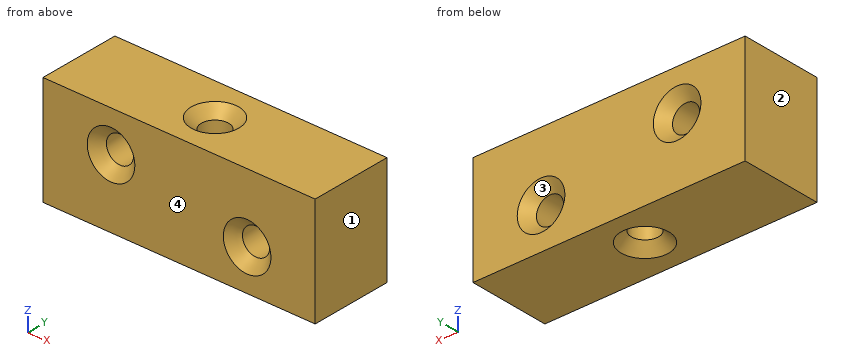
```python
from build123d import *

# Parameters (mm, degrees)
F0_W     = 40
F0_H     = 16
F0_R     = 2
F1_DEPTH = 12
F2_R     = 2
F3_DEPTH = 16.001
F4_SIZE  = 1.5


with BuildPart() as f1:
    # F0 (on Front) → F1 (new body)
    with BuildSketch(Plane.XZ):
        Rectangle(F0_W, F0_H)
        with Locations((10, -2)):
            Circle(F0_R, mode=Mode.SUBTRACT)
        with Locations((-10, 2)):
            Circle(F0_R, mode=Mode.SUBTRACT)
    extrude(amount=-F1_DEPTH)

    # F2 (on face) → F3 (cut, through all)
    with BuildSketch(Plane.XY.offset(8)):
        with Locations((0, 6)):
            Circle(F2_R)
    extrude(amount=-F3_DEPTH, mode=Mode.SUBTRACT)

    # F4
    f4_edges = [f1.edges().sort_by_distance(p)[0] for p in [
        (-12, 12, 2),
        (8, 12, -2),
        (-12, 0, 2),
        (8, 0, -2),
        (-2, 6, 8),
        (-2, 6, -8),
    ]]
    chamfer(f4_edges, length=F4_SIZE)


solid = f1.part
```
Can you work these out from the model? Positions are in its coordinate system, mm. Face numbers are marked on the shaded views. Coordinates: 2 decimals unless noted, no trailing zeros. Order: outer loops, then holes, each group sorted by start corner. A loop starts at its lowest first (then second) coordinate and runs counter-clockwise, first axis right, second up.
1. I need wall thicknesses on line 1 (Z direction, x = -10, y = 3.75); line 2 (Z direction, x = 10, y = 4.5); line 3 (X direction, y = 5.5, z = -2.5). Which ranges of each line are inside material? Lowest first, please.
2. If we section it at A-A (y = 6): Please give me the cut outline in (x, z), then the cut area to 3 significant figures.
3. If we section it at D-D (z = 6): Please give me the cut outline in (x, y), then the cut area to 3 significant figures.
4. Thinking about a two-plate mould opening in X: for the marked faces 1, 2, 3 and 4, which applies, +X half, -X half, draft (parallel to the pull), parting line (faces both ways), or undercut?
5. I'm going to push flat-ended pins straight in: pin 1 (8 mm diameter, centred on x = 14, z = 5.5, fed in from -Y); pin 2 (5 mm diameter, centred on x = -10, z = 2, fed in from +Y). Where does each tip first touch, or does it pass through?
6. If we section it at B-B (x = 0): Please give me the cut outline in (y, z).
7. If we section it at C-C (z = -2): Please give me the cut outline in (x, y), then the cut area to 3 significant figures.
Entries:
1. line 1: z = -8 to 0, 4 to 8
1. line 2: z = -8 to -4, 0 to 8
1. line 3: x = -20 to -1.94, 1.94 to 8.06, 11.94 to 20
2. outline: (-20, -8) - (-3.5, -8) - (-2, -6.5) - (-2, 6.5) - (-3.5, 8) - (-20, 8) - close; (2, -6.5) - (3.5, -8) - (20, -8) - (20, 8) - (3.5, 8) - (2, 6.5) - close; hole circle Ø4 at (-10, 2); hole circle Ø4 at (10, -2)
2. area: 546 mm2
3. outline: (-20, 0) - (20, 0) - (20, 12) - (-20, 12) - close; hole circle Ø4 at (0, 6)
3. area: 467 mm2
4. face 1: +X half
4. face 2: -X half
4. face 3: undercut
4. face 4: draft
5. pin 1: stops at y = 0
5. pin 2: stops at y = 11
6. outline: (0, -8) - (2.5, -8) - (4, -6.5) - (4, 6.5) - (2.5, 8) - (0, 8) - close; (8, -6.5) - (9.5, -8) - (12, -8) - (12, 8) - (9.5, 8) - (8, 6.5) - close
7. outline: (-20, 0) - (6.5, 0) - (8, 1.5) - (8, 10.5) - (6.5, 12) - (-20, 12) - close; (12, 1.5) - (13.5, 0) - (20, 0) - (20, 12) - (13.5, 12) - (12, 10.5) - close; hole circle Ø4 at (0, 6)
7. area: 415 mm2
